Geometry: final body of the model. Coordinates: model frame, mm. Face numbers are marked on the shaded views. A direction names the side the tool comes from. Round coordinates to 2 decimals unless told otherwise and drop trailing zeros. Loops run counter-clockwise (first coordinate to the right, second up) from the corner with the lowest first, then second, coordinate; pieces in that order, holes last. Notation, with made-up numbers: (42, 86.5) - (54, 86.5) arc R23 cw to (54, 107.5) - close; hole circle Ø4 at (39, -4.75). An arc over 180 degrees is marked (long way). Use CSV: the item, a comma, the result in double quotes.
from build123d import *

# Parameters (mm, degrees)
F0_R     = 27.654289
F0_R_2   = 31.789504
F1_DEPTH = 76.2
F3_R     = 22.213723
F4_DEPTH = 25.4
F5_DEPTH = 157.734


with BuildPart() as f1:
    # F0 (on Top) → F1 (new body)
    with BuildSketch(Plane.XY):
        Polygon((117.248647, 64.562328), (-111.418605, 64.562328), (-111.418605, -51.62568), (-156.081602, -51.62568), (-156.081602, -77.738054), (-79.898089, -77.738054), (-79.898089, -60.891561), (117.248647, -60.891561), align=None)
        with Locations((-66.341519, -20.300921)):
            Circle(F0_R, mode=Mode.SUBTRACT)
        with Locations((62.335916, 17.92543)):
            Circle(F0_R_2, mode=Mode.SUBTRACT)
    extrude(amount=F1_DEPTH)

    # F3 (on face) → F4 (cut)
    with BuildSketch(Plane(origin=(0, 64.562328, 0), x_dir=(-1, 0, 0), z_dir=(0, 1, 0))):
        with Locations((-3.41973, 36.301557)):
            Circle(F3_R)
    extrude(amount=-F4_DEPTH, mode=Mode.SUBTRACT)

    # F2 (on face) → F5 (cut)
    with BuildSketch(Plane.XZ.offset(77.738054)):
        Polygon((-131.27912, 11.703248), (-89.60872, 42.351646), (-136.986211, 63.115072), align=None)
    extrude(amount=-F5_DEPTH, mode=Mode.SUBTRACT)


solid = f1.part
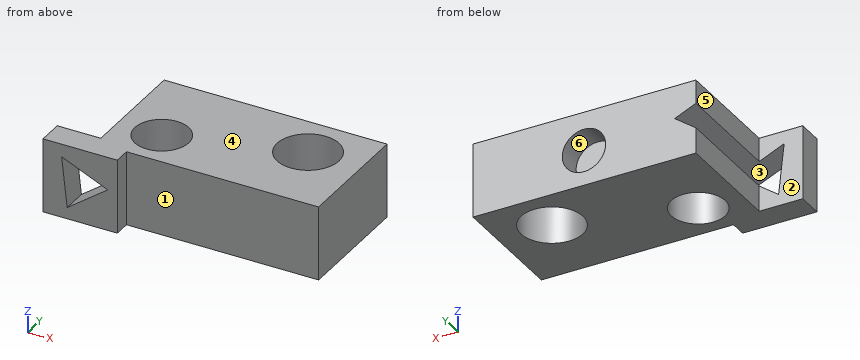
Item 1: Material intervals for line 1 (Z direction, x = 4, y = 41.5); line 2 (X direction, y = 47, z = 55); line 3 (X direction, y = -4, z = 58.5), sorted ascending.
Final values:
line 1,"z = 0 to 14.1, 58.51 to 76.2"
line 2,"x = -111.42 to -8.57, 15.41 to 49.48, 75.19 to 117.25"
line 3,"x = -111.42 to -88.68, -44 to 39.32, 85.35 to 117.25"
Item 2: Pin query (flat end, axial travel): P1, Ø12, axis at y = 20.5, z = 59, coming from the -X side; P2, Ø13.5, axis at x = -130.5, z = 40, coming from the +Y side; P3, Ø18.5, axis at y = -67, z = 39, coming from the +X side; P4, Ø2, axis at x = 56, z = 30, coming from the -Y side. Return the tip coordinate at first contact, or that it passes through.
Final values:
P1,"stops at x = -111.42"
P2,"stops at y = -51.63"
P3,"stops at x = 117.25"
P4,"stops at y = -60.89"
Item 3: Section D-D on y = 23. Return the cut outline in (x, z), plus the area to 3 significant figures.
Final values:
outline,"(-111.42, 0) - (30.95, 0) - (30.95, 76.2) - (-111.42, 76.2) - (-111.42, 51.91) - (-89.61, 42.35) - (-111.42, 26.31) - close; (93.72, 0) - (117.25, 0) - (117.25, 76.2) - (93.72, 76.2) - close"
area,"12,400 mm²"
Item 4: Section B-B on y = -58. Return the cut outline in (x, z).
Final values:
outline,"(-156.08, 0) - (117.25, 0) - (117.25, 76.2) - (-156.08, 76.2) - close; hole (-136.99, 63.12) - (-131.28, 11.7) - (-89.61, 42.35) - close"
Item 5: Mould query, pull axis Z, two halves, no side actions, for the marked faces 4, 5 and 6. Classes: released by +Z, released by -Z, zero draft, split by the parting line, or undercut.
Final values:
face 4,"released by +Z"
face 5,"zero draft"
face 6,"undercut"
Item 6: Reachability of the marked faces 1, 2 and 3 from +Z, -Z, +X, -X, +Y, -Y: full face, straight path, thin tool, end or side. Return the list, or none.
Final values:
face 1,"+Z, -Z, +X, -Y"
face 2,"+Z, -Z, -X, +Y"
face 3,"+Y, -Y"
Item 7: Section A-A on z = 45.5. Return the cut outline in (x, y).
Final values:
outline,"(-156.08, -77.74) - (-135.03, -77.74) - (-135.03, -51.63) - (-156.08, -51.63) - close; (-96.79, -77.74) - (-79.9, -77.74) - (-79.9, -60.89) - (117.25, -60.89) - (117.25, 64.56) - (23.64, 64.56) - (23.64, 39.16) - (-16.8, 39.16) - (-16.8, 64.56) - (-96.79, 64.56) - close; hole circle Ø55.31 at (-66.34, -20.3); hole circle Ø63.58 at (62.34, 17.93)"
Item 8: Section C-C on x = -114.5. Return the cut outline in (y, z), plus the area to 3 significant figures.
Final values:
outline,"(-77.74, 0) - (-51.63, 0) - (-51.63, 24.04) - (-77.74, 24.04) - close; (-77.74, 53.26) - (-51.63, 53.26) - (-51.63, 76.2) - (-77.74, 76.2) - close"
area,"1,230 mm²"
